```python
from build123d import *

# Parameters (mm, degrees)
SKETCH_W     = 10.67
SKETCH_H     = 9.4
PAD_DEPTH    = 4.7
SKETCH001_R  = 0.75
PAD001_DEPTH = 3.5
SKETCH002_R  = 0.35
PAD002_DEPTH = 10
SKETCH003_W  = 10.67
SKETCH003_H  = 0.55
PAD003_DEPTH = 6.5
SKETCH004_R  = 2
POCKET_DEPTH = 5


with BuildPart() as part:
    # Sketch → Pad (new body)
    with BuildSketch(Plane.XY):
        with Locations((5.335, 4.7)):
            Rectangle(SKETCH_W, SKETCH_H)
    extrude(amount=PAD_DEPTH)

    # Sketch001 → Pad001 (new body)
    with BuildSketch(Plane.XZ):
        with Locations((2.795, 2.6)):
            Circle(SKETCH001_R)
        with Locations((5.335, 2.6)):
            Circle(SKETCH001_R)
        with Locations((7.875, 2.6)):
            Circle(SKETCH001_R)
    extrude(amount=PAD001_DEPTH)

    # Sketch002 → Pad002 (new body)
    with BuildSketch(Plane.XZ.offset(3.5)):
        with Locations((2.795, 2.6)):
            Circle(SKETCH002_R)
        with Locations((5.335, 2.6)):
            Circle(SKETCH002_R)
        with Locations((7.875, 2.6)):
            Circle(SKETCH002_R)
    extrude(amount=PAD002_DEPTH)

    # Sketch003 → Pad003 (new body)
    with BuildSketch(Plane(origin=(0, 9.4, 0), x_dir=(-1, 0, 0), z_dir=(0, 1, 0))):
        with Locations((-5.335, 0.275)):
            Rectangle(SKETCH003_W, SKETCH003_H)
    extrude(amount=PAD003_DEPTH)

    # Sketch004 → Pocket (cut)
    with BuildSketch(Plane.XY.offset(0.55)):
        with Locations((5.335, 12.9)):
            Circle(SKETCH004_R)
    extrude(amount=-POCKET_DEPTH, mode=Mode.SUBTRACT)


solid = part.part
```
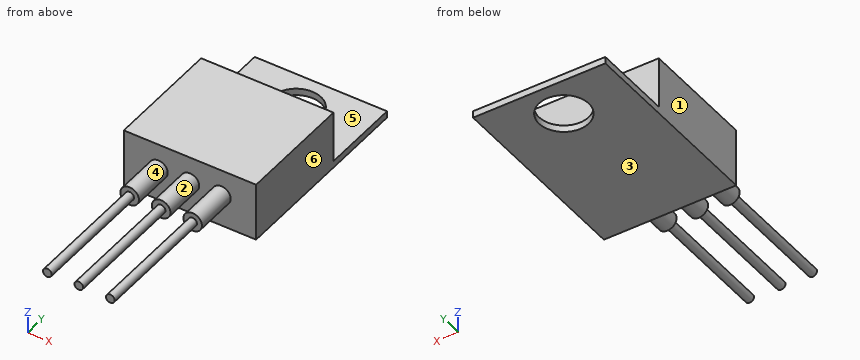
Work out the finished part from the listing and answer in its coordinate system (mm). Face numbers are marked on the shaded views. A direction names the side the tool comes from. Round coordinates to 2 decimals unless told otherwise and drop trailing zeros. Write each loop counter-clockwise with the first axis right and the second up, starting at its lowest first coordinate (ties: lowest second). Pieces come first, ordered by that corner, then holes.
1) A cutting plane is placed at B-B on z = 2.6. Determine the outline of the cut face in (x, y) (3 decimals), and give its area (3 significant figures).
2) Flat-ended cylindrical pins translate along their axes: P1, Ø5, axis at x = 6.5, y = 13.5, coming from the +Z side; P2, Ø1.5, axis at x = 2.5, z = 4, coming from the -Y side; P3, Ø3, axis at x = 5.335, y = 12.9, coming from the -Z side; P4, Ø5, axis at x = 9.5, y = 9, coming from the -Z side. Find the tip coordinate at first contact, or state that the pin passes through.
3) A cutting plane is placed at A-A on y = 12.9. Determine the outline of the cut face in (x, z) (3 decimals), and give its area (3 significant figures).
4) A cutting plane is placed at D-D on x = 10. Determine the outline of the cut face in (y, z), and give its area (3 significant figures).
5) Determine the mould class of the marked faces 1, 2 and 3 for opening direction X: pulls with the +X half, pulls with the -X half, needs draft (parallel to the pull), parting line crosses it, or undercut.
6) Consider probe 1 along Z at (x, y) = (3.5, 11.75); probe 2 along Y at (x, z) = (8, 3.8); probe 3 along Y at (x, z) = (4.5, 0.5). Determine where each line is inside the solid, lowest interval first.
7) A cutting plane is placed at C-C on y = -0.5. Determine the outline of the cut face in (x, z) (3 decimals), and give its area (3 significant figures).
8) Which of the six approach directions +Z, -Z, +X, -X, +Y, -Y give full straight-line access (tool end or side, diameter ignored) to the marked faces 4, 5 and 6?
Entries:
1. outline: (0, 0) - (2.045, 0) - (2.045, -3.5) - (2.445, -3.5) - (2.445, -13.5) - (3.145, -13.5) - (3.145, -3.5) - (3.545, -3.5) - (3.545, 0) - (4.585, 0) - (4.585, -3.5) - (4.985, -3.5) - (4.985, -13.5) - (5.685, -13.5) - (5.685, -3.5) - (6.085, -3.5) - (6.085, 0) - (7.125, 0) - (7.125, -3.5) - (7.525, -3.5) - (7.525, -13.5) - (8.225, -13.5) - (8.225, -3.5) - (8.625, -3.5) - (8.625, 0) - (10.67, 0) - (10.67, 9.4) - (0, 9.4) - close
1. area: 137 mm2
2. P1: stops at z = 0.55
2. P2: stops at y = -3.5
2. P3: passes through
2. P4: stops at z = 0
3. outline: (0, 0) - (3.335, 0) - (3.335, 0.55) - (0, 0.55) - close; (7.335, 0) - (10.67, 0) - (10.67, 0.55) - (7.335, 0.55) - close
3. area: 3.67 mm2
4. outline: (0, 0) - (15.9, 0) - (15.9, 0.55) - (9.4, 0.55) - (9.4, 4.7) - (0, 4.7) - close
4. area: 47.8 mm2
5. face 1: pulls with the -X half
5. face 2: undercut
5. face 3: needs draft
6. probe 1: z = 0 to 0.55
6. probe 2: y = 0 to 9.4
6. probe 3: y = 0 to 11.08, 14.72 to 15.9
7. outline: circle Ø1.5 at (2.795, 2.6); circle Ø1.5 at (5.335, 2.6); circle Ø1.5 at (7.875, 2.6)
7. area: 5.30 mm2
8. face 4: -Y
8. face 5: +Z, +X, -X, +Y
8. face 6: +Z, -Z, +X, +Y, -Y
